from build123d import *

# Parameters (mm, degrees)
SKETCH1_R           = 5
BOSS_EXTRUDE1_DEPTH = 6


with BuildPart() as part:
    # Sketch1 → Boss-Extrude1 (new body)
    with BuildSketch(Plane.XY):
        with BuildLine():
            Line((9.999881276, -0.048728438), (8.050720605, -400.048728438))
            ThreePointArc((8.050720605, -400.048728438), (-1.99788911, -409.999881276), (-11.949041948, -399.951271562))
            Line((-11.949041948, -399.951271562), (-9.999881276, 0.048728438))
            ThreePointArc((-9.999881276, 0.048728438), (0.048728438, 9.999881276), (9.999881276, -0.048728438))
        make_face()
        with Locations((-1.949160671, -400)):
            Circle(SKETCH1_R, mode=Mode.SUBTRACT)
        Circle(SKETCH1_R, mode=Mode.SUBTRACT)
    boss_extrude1 = extrude(amount=BOSS_EXTRUDE1_DEPTH)

    # Mirror1: Boss-Extrude1 across plane
    add(boss_extrude1.mirror(Plane.XY))


solid = part.part
Could you check a few things on this model? Use its own coordinates, in mm. Give positions to 0.01 mm unless a question says otherwise; leave off trailing zeros. Loops run counter-clockwise (first coordinate to the right, second up) from the corner with the lowest first, then second, coordinate; pieces in that order, holes last. Notation, with made-up numbers: (-34.75, -18) -> (-12.75, -18) arc R32 ccw to (-12.75, 12) -> close; hole circle Ø10 at (40, 79). An arc over 180 degrees is marked (long way). Return JSON: item names as keys, results as strings.
Item 1: I need wall thicknesses on L1, parallel to X at y = -400, z = -2.75; L2, parallel to Y at x = -0.25, z = -4.5; L3, parallel to Y at x = -2.75, z = 1. Which ranges of each line are inside material? Lowest first, please. Write a range as from..to.
Geometry results:
{"L1": "x = -11.95..-6.95, 3.05..8.05", "L2": "y = -409.85..-404.7, -395.3..-4.99, 4.99..10", "L3": "y = -409.97..-404.94, -395.06..-4.18, 4.18..9.61"}
Item 2: If we section it at B-B on z = 3: List the corners of the cut face in (x, y) for me.
Geometry results:
{"outline": "(-11.95, -399.95) arc R10 ccw to (8.05, -400.05) -> (10, -0.05) arc R10 ccw to (-10, 0.05) -> close; hole circle Ø10 at (-1.95, -400); hole circle Ø10 at (0, 0)"}
Item 3: We'd pull the mould along X, two halves only. Please class faces 1 (the cylindrical face through (-1.08, -4.88, -0.08)), 2 (the cylindrical face through (-2, -410, 0)), 3 (the cylindrical face through (-2.6, -395.043, -0.084)), 4 (the flat face through (-1, -197, -6)): +X half, -X half, draft (parallel to the pull), parting line (faces both ways), or undercut.
Geometry results:
{"face 1": "undercut", "face 2": "parting line", "face 3": "undercut", "face 4": "draft"}
Item 4: If we section it at C-C on y = -219.5: List the corners of the cut face in (x, z) for me, plus the area to 3 significant figures.
Geometry results:
{"outline": "(-11.07, -6) -> (8.93, -6) -> (8.93, 6) -> (-11.07, 6) -> close", "area": "240 mm²"}
Item 5: I'm going to push flat-ended pins straight in: pin 1 (13 mm diameter, centred on x = 0, y = 0, fed in from -Z); pin 2 (2 mm diameter, centred on y = -171, z = -4, fed in from +X); pin 3 (6 mm diameter, centred on x = -1.95, y = -400, fed in from +Z); pin 4 (3 mm diameter, centred on x = -5, z = -4.5, fed in from +Y). Where does each tip first touch, or does it pass through?
Geometry results:
{"pin 1": "stops at z = -6", "pin 2": "stops at x = 9.17", "pin 3": "passes through", "pin 4": "stops at y = 9.37"}
Item 6: If we section it at A-A on x = -1.25: List the corners of the cut face in (y, z) for me.
Geometry results:
{"outline": "(-409.98, -6) -> (-404.95, -6) -> (-404.95, 6) -> (-409.98, 6) -> close; (-395.05, -6) -> (-4.84, -6) -> (-4.84, 6) -> (-395.05, 6) -> close; (4.84, -6) -> (9.92, -6) -> (9.92, 6) -> (4.84, 6) -> close"}
